Autodesk Inventor part; units mm, degrees
ref_plane "YZ Plane" through (0, 0, 0) normal (1, 0, 0) x (0, 1, 0)
ref_plane "XZ Plane" through (0, 0, 0) normal (0, 1, 0) x (-1, 0, 0)
ref_plane "XY Plane" through (0, 0, 0) normal (0, 0, 1) x (1, 0, 0)
sketch "Sketch1" plane through (0, 0, 0) normal (1, 0, 0) x (0, 1, 0)
  line L0 (-0.5, 45) -> (0.5, 45)
  line L1 (0.5, 45) -> (0.5, -45)
  line L2 (0.5, -45) -> (-0.5, -45)
  line L3 (-0.5, -45) -> (-0.5, 45)
  line L4 (-0.5, 45) -> (0.5, -45) construction
  line L5 (0.5, 45) -> (-0.5, -45) construction
  line L6 (-0.5, 45) -> (-5.5, 45)
  line L7 (-5.5, 45) -> (-5.5, 50)
  line L8 (-5.5, 50) -> (-10.5, 50)
  line L9 (-10.5, 50) -> (-10.5, 55)
  arc A0 (-0.5, 45) -> (-5.5, 50) centre (-5.5, 45) ccw
  arc A1 (-10.5, 55) -> (-5.5, 50) centre (-5.5, 55) ccw
  line L10 (-5.5, 50) -> (-5.5, 51)
  arc A2 (0.5, 45) -> (-5.5, 51) centre (-5.5, 45) ccw
  line L11 (-10.5, 55) -> (-9.5, 55)
  line L12 (-10.5, 55) -> (-9.5, 55)
  line L13 (-9.5, 55) -> (-9.5, 165)
  line L14 (-9.5, 165) -> (-10.5, 165)
  line L15 (-10.5, 165) -> (-10.5, 55)
  arc A3 (-9.5, 55) -> (-5.5, 51) centre (-5.5, 55) ccw
  point P0 (0, 0)
  dimension "d0" = 1
  dimension "d1" = 90
  dimension "d2" = 5
  dimension "d3" = 5
  dimension "d4" = 5
  dimension "d5" = 5
  dimension "d6" = 5
  dimension "d7" = 5
  dimension "d8" = 1
  dimension "d9" = 6
  dimension "d10" = 1
  dimension "d12" = 1
  dimension "d13" = 110
  dimension "d14" = 4
extrude "Extrusion1" add sketch "Sketch1" along normal blind 70 contours A0 L10 A2 L0 | L0 L1 L2 L3 | A1 L11 A3 L10 | L15 L14 L13 L11
sketch "Sketch2" plane through (0, 0.5, 45) normal (0, 1, 0) x (1, 0, 0)
  circle A0 centre (5, 85) radius 1.5
  circle A1 centre (65, 85) radius 1.5
  line L0 (0, 90) -> (70, 90)
  line L1 (70, 90) -> (70, 0)
  line L2 (0, 90) -> (0, 0)
  point P0 (0, 45)
  dimension "d17" = 3
  dimension "d18" = 3
  dimension "d19" = 5
  dimension "d20" = 5
  dimension "d21" = 5
  dimension "d22" = 5
extrude "Extrusion2" cut sketch "Sketch2" against normal up to next
sketch "Sketch3" plane through (0, -9.5, 165) normal (0, 1, 0) x (1, 0, 0)
  circle A0 centre (5, 100) radius 1.5
  circle A1 centre (65, 100) radius 1.5
  line L0 (0, 110) -> (70, 110)
  line L1 (70, 110) -> (70, 0)
  line L2 (0, 110) -> (0, 0)
  point P0 (0, 165)
  dimension "d25" = 3
  dimension "d26" = 3
  dimension "d27" = 10
  dimension "d28" = 5
  dimension "d29" = 10
  dimension "d30" = 5
extrude "Extrusion3" cut sketch "Sketch3" against normal up to next
sketch "Sketch4" plane through (0, -10.5, 165) normal (0, 0, 1) x (1, 0, 0)
  line L0 (0, 0) -> (70, 0)
  line L1 (0, 0) -> (70, 0)
  line L2 (70, 0) -> (70, 1)
  line L3 (70, 1) -> (0, 1)
  line L4 (0, 1) -> (0, 0)
  point P0 (0, 10.5)
extrude "Extrusion4" add sketch "Sketch4" along normal blind 5.5
sketch "Sketch5" plane through (0, -9.5, 55) normal (0, 1, 0) x (1, 0, 0)
  line L0 (70, -115.5) -> (0, -115.5)
  line L1 (35, -115.5) -> (35, -110.5)
  circle A0 centre (35, -110.5) radius 1.5
  point P0 (0, 55)
  dimension "d35" = 5
  dimension "d36" = 3
extrude "Extrusion5" cut sketch "Sketch5" against normal up to next
sketch "Sketch6" plane through (0, -9.5, 55) normal (0, 1, 0) x (1, 0, 0)
  line L0 (70, -115.5) -> (0, -115.5)
  line L1 (35, -115.5) -> (60, -115.5)
  line L2 (35, -115.5) -> (10, -115.5)
  line L3 (0, -115.5) -> (0, -65.5)
  line L4 (0, 0) -> (0, -115.5)
  line L5 (70, -115.5) -> (70, -65.5)
  line L6 (70, 0) -> (70, -115.5)
  line L7 (70, -65.5) -> (60, -115.5)
  line L8 (0, -65.5) -> (10, -115.5)
  line L9 (10, -115.5) -> (0, -115.5)
  line L10 (60, -115.5) -> (70, -115.5)
  point P0 (0, 55)
  dimension "d39" = 25
  dimension "d40" = 25
  dimension "d41" = 50
  dimension "d42" = 50
extrude "Extrusion6" cut sketch "Sketch6" against normal up to next
properties part number "cover" material "PET Plastic"
Input: part model. Units: mm. Frame: model coordinates. A direction names the side the tool comes from. Coordinates: 2 decimals unless noted, no trailing zeros. Loops run counter-clockwise (first coordinate to the right, second up) from the corner with the lowest first, then second, coordinate; pieces in that order, holes last. Notation, with made-up numbers: (52.25, -5.75) -> (97.25, -5.75) arc R27 ccw to (97.25, 14.25) -> close; hole circle Ø6 at (72.5, -33.5). An arc over 180 degrees is marked (long way). One line per item, written item: value.
(1) Set-up query: faces 1 (the face through (35, 0.5, 1)), 2 (the face through (35, -9.5, 112)), 3 (the face through (35, -0.5, -1)). Return all of +Z, -Z, +X, -X, +Y, -Y with unobstructed straight access to the full face (end or side cutting, diameter ignored); none if empty.
Answer below:
face 1: +Z, -Z, +X, -X, +Y
face 2: +Z, +X, -X, +Y
face 3: -Z, +X, -X, -Y
(2) Cut plane B-B (z = 70.5). Output: boundary loops of the cut face in (x, y).
Answer below:
outline: (0, -10.5) -> (70, -10.5) -> (70, -9.5) -> (0, -9.5) -> close
(3) Cut plane A-A (x = 27.5). Output: boundary loops of the cut face in (y, z), then the cut area to 3 significant figures.
Answer below:
outline: (-10.5, 55) arc R5 ccw to (-5.5, 50) arc R5 cw to (-0.5, 45) -> (-0.5, -45) -> (0.5, -45) -> (0.5, 45) arc R6 ccw to (-5.5, 51) arc R4 cw to (-9.5, 55) -> (-9.5, 170.5) -> (-10.5, 170.5) -> close
area: 221 mm2
(4) Pin query (flat end, axial travel): pin 1 Ø4 at (x, z) = (65, -40) entering from -Y; pin 2 Ø1.5 at (x, y) = (18.5, -9) entering from -Z; pin 3 Ø5 at (x, z) = (14, 118) entering from +Y. Return the tip coordinate at first contact, or that it passes through.
Answer below:
pin 1: stops at y = -0.5
pin 2: stops at z = 50.82
pin 3: stops at y = -9.5
(5) Ray query, line 1 along X through (y, z) = (-10.2, 65); line 2 along Y through (x, z) = (33.5, 73.5); line 3 along Z through (x, y) = (10, -5). Return the intervals inside material, ascending.
Answer below:
line 1: x = 0 to 3.5, 6.5 to 63.5, 66.5 to 70
line 2: y = -10.5 to -9.5
line 3: z = 49.97 to 50.98
(6) Cut plane C-C (y = -3.5). Output: boundary loops of the cut face in (x, z).
Answer below:
outline: (0, 49.58) -> (70, 49.58) -> (70, 50.66) -> (0, 50.66) -> close
